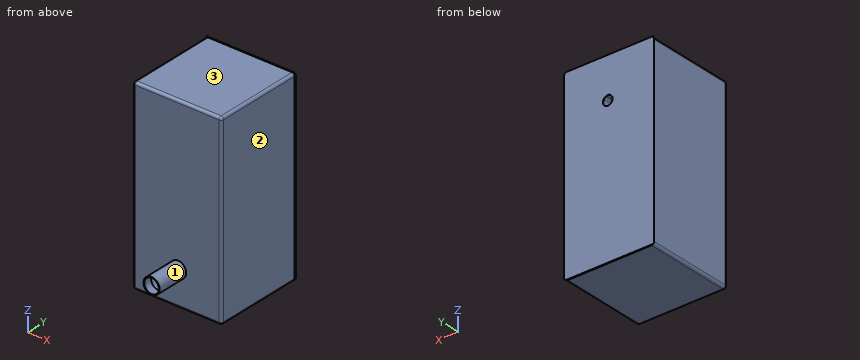
Autodesk Inventor part; units mm, degrees
ref_plane "YZ Plane" through (0, 0, 0) normal (1, 0, 0) x (0, 1, 0)
ref_plane "XZ Plane" through (0, 0, 0) normal (0, 1, 0) x (-1, 0, 0)
ref_plane "XY Plane" through (0, 0, 0) normal (0, 0, 1) x (1, 0, 0)
sketch "Sketch1" plane through (0, 0, 0) normal (0, 0, 1) x (1, 0, 0)
  line L0 (0, 0) -> (-110, 0)
  line L1 (-110, 0) -> (-110, 110)
  line L2 (-110, 110) -> (0, 110)
  line L3 (0, 110) -> (0, 0)
  dimension "d0" = 110
  dimension "d1" = 110
extrude "Extrusion1" add sketch "Sketch1" along normal blind 230
fillet "Fillet2" radius 3.175 8 edges at (-110, 55, 230) (0, 55, 230) (-55, 0, 230) (-110, 0, 115) (0, 0, 115) (0, 55, 0) (-55, 0, 0) (-110, 55, 0)
shell "Shell1" thickness 0.5 removed faces 1 at (-36.6667, 110, 77.725)
sketch "Sketch2" plane through (-106.825, 110, 0) normal (0, 1, 0) x (1, 0, 0)
  line L0 (-2.54, -230.635) -> (107.9059, -230.635)
  line L1 (107.9059, -230.635) -> (107.9059, -0.635)
  line L2 (107.9059, -0.635) -> (-2.54, -0.635)
  line L3 (-2.54, -0.635) -> (-2.54, -230.635)
  point P0 (106.825, 0)
  point P1 (0, -229.5)
  point P2 (103.65, -3.175)
  dimension "d11" = 230
extrude "Extrusion2" add sketch "Sketch2" along normal blind 0.5
fillet "Fillet4" radius 3.175 2 edges at (1.0809, 110.25, 230.635) (1.0809, 110.25, 0.635)
sketch "Sketch3" plane through (-106.825, 110.5, 0) normal (0, 1, 0) x (1, 0, 0)
  point P0 (106.825, 0)
  point P1 (53.8726, -180.2016)
hole "Hole1" at (-52.9524, 110.5, 180.2016) direction (0, -1, 0) diameter 12 depth 10 tip angle 118
sketch "Sketch4" plane through (-106.825, 0, 3.175) normal (0, -1, 0) x (1, 0, 0)
  point P0 (106.825, -3.175)
  point P1 (53.016, 39.15)
hole "Hole2" at (-53.809, 0, 42.325) direction (0, 1, 0) diameter 18 depth 10 tip angle 118
sketch "Sketch5" plane through (-106.825, 0, 3.175) normal (0, -1, 0) x (1, 0, 0)
  circle A0 centre (53.016, 39.15) radius 9
  circle A1 centre (53.016, 39.15) radius 10
  point P0 (106.825, -3.175)
  dimension "d27" = 20
extrude "Extrusion3" add sketch "Sketch5" along normal blind 40 contours A0 | A1
sketch "Sketch6" plane through (-53.809, -40, 42.325) normal (0, -1, 0) x (1, 0, 0)
  point P0 (53.809, -42.325)
  point P1 (0.11, 0.0758)
hole "Hole3" at (-53.6991, -40, 42.4008) direction (0, 1, 0) diameter 18 depth 10 tip angle 118
properties part number "oil_water_separator"
Source: CAD feature listing. Evaluate the final solid. Frame: model axes, mm. Face numbers are marked on the shaded views. A direction names the side the tool comes from. Round coordinates to 2 decimals unless told otherwise and drop trailing zeros. Write each loop counter-clockwise with the first axis right and the second up, starting at its lowest first coordinate (ties: lowest second). Pieces come first, ordered by that corner, then holes. Notation, with made-up numbers: M 22,70 L 46,70 A32 cw 46,97 Z; hole C 78.5,-33.75 d4. An arc over 180 degrees is marked long. Answer as a JSON object with one key per item and string values. Group by question number.
(1) First-contact query: pin 1 (4 mm diameter, centred on x = -34.5, z = 190.5, fed in from -Y); pin 2 (12 mm diameter, centred on y = -1.5, z = 76.5, fed in from +X); pin 3 (7 mm diameter, centred on x = -52.95, z = 180.2, fed in from +Y); pin 4 (10 mm diameter, centred on x = -49.5, y = 8.5, fed in from -Z). Flat tips, straight axial feed; report the tip coordinate or a pass-through.
(2) Section query C-C on z = 190. Output: boundary loops of the cut face in (x, y) (3 decimals), then the cut area to 3 significant figures.
(3) Section query D-D on y = -9.5. Output: boundary loops of the cut face in (x, z) (3 decimals).
(4) Reachability of the marked faces 1, 2 and 3 from +Z, -Z, +X, -X, +Y, -Y: full face, straight path, thin tool, end or side. Return the list, or none.
(5) Section query B-B on x = -91.5. Output: boundary loops of the cut face in (y, z) (3 decimals), then the cut area to 3 significant figures.
(6) Ray query, line 1 (Y direction, x = -103.5, z = 68); line 2 (Z direction, x = -94.5, y = 100); line 3 (X direction, y = 73.5, z = 196). Return the intervals inside material, ascending. Write a range as [from, to].
(7) Section query A-A on y = 44.5. Output: boundary loops of the cut face in (x, z) (3 decimals), then the cut area to 3 significant figures.
Computed values:
{
 "1": {"pin 1": "y = 0", "pin 2": "x = 0", "pin 3": "y = 0.5", "pin 4": "z = 0"},
 "2": {"outline": "M -110,3.175 A3.175 ccw -106.825,0 L -3.175,0 A3.175 ccw 0,3.175 L 0,110 L 1.081,110 L 1.081,110.5 L -109.365,110.5 L -109.365,110 L -0.5,110 L -0.5,3.175 A2.675 cw -3.175,0.5 L -106.825,0.5 A2.675 cw -109.5,3.175 L -109.5,110 L -110,110 Z", "area": "218 mm^2"},
 "3": {"outline": "C -53.809,42.325 d20"},
 "4": {"face 1": "-Y", "face 2": "+Z, -Z, +X, -Y", "face 3": "+Z, +X, -X, -Y"},
 "5": {"outline": "M 0,3.175 A3.175 ccw 3.175,0 L 110,0 L 110,0.5 L 3.175,0.5 A2.675 cw 0.5,3.175 L 0.5,226.825 A2.675 cw 3.175,229.5 L 110,229.5 L 110,0.635 L 110.5,0.635 L 110.5,230.635 L 110,230.635 L 110,230 L 3.175,230 A3.175 ccw 0,226.825 Z", "area": "338 mm^2"},
 "6": {"line 1": "[0, 0.5], [110, 110.5]", "line 2": "[0, 0.5], [229.5, 230]", "line 3": "[-110, -109.5], [-0.5, 0]"},
 "7": {"outline": "M -110,3.175 A3.175 ccw -106.825,0 L -3.175,0 A3.175 ccw 0,3.175 L 0,226.825 A3.175 ccw -3.175,230 L -106.825,230 A3.175 ccw -110,226.825 Z; hole M -109.5,3.175 A2.675 ccw -106.825,0.5 L -3.175,0.5 A2.675 ccw -0.5,3.175 L -0.5,226.825 A2.675 ccw -3.175,229.5 L -106.825,229.5 A2.675 ccw -109.5,226.825 Z", "area": "336 mm^2"}
}
